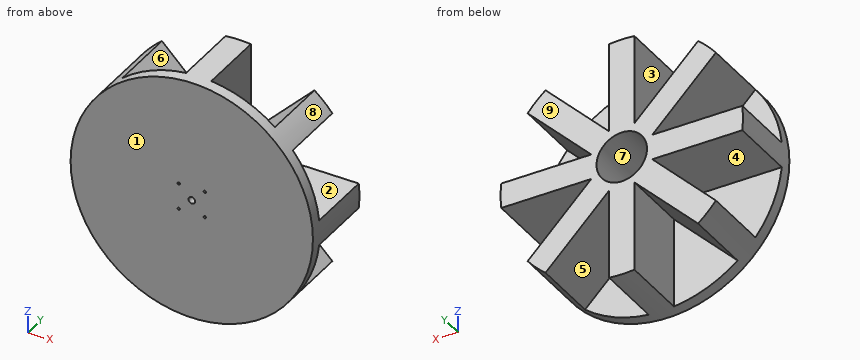
```python
from build123d import *

# Parameters (mm, degrees)
SKETCH1_R           = 144
BOSS_EXTRUDE1_DEPTH = 94
CUT_EXTRUDE1_DEPTH  = 80
SKETCH3_R           = 4
CUT_EXTRUDE2_DEPTH  = 20
CUT_EXTRUDE3_REACH  = 96
SKETCH4_R           = 1.4
SKETCH5_R           = 30
CUT_EXTRUDE4_DEPTH  = 80


with BuildPart() as part:
    # Sketch1 → Boss-Extrude1 (new body)
    with BuildSketch(Plane(origin=(0, 0, 0), x_dir=(1, 0, 0), z_dir=(0, 1, 0))):
        Circle(SKETCH1_R)
    extrude(amount=BOSS_EXTRUDE1_DEPTH)

    # Sketch2 → Cut-Extrude1 (cut)
    with BuildSketch(Plane(origin=(0, 94, 0), x_dir=(1, 0, 0), z_dir=(0, 1, 0))):
        with BuildLine():
            Line((-15, 36.213203436), (-15, 143.216619147))
            ThreePointArc((-15, 143.216619147), (-55.106414261, 133.038652682), (-90.66284086, 111.876044296))
            Line((-90.66284086, 111.876044296), (-15, 36.213203436))
        make_face()
        with BuildLine():
            Line((15, 36.213203436), (90.66284086, 111.876044296))
            ThreePointArc((90.66284086, 111.876044296), (55.106414261, 133.038652682), (15, 143.216619147))
            Line((15, 143.216619147), (15, 36.213203436))
        make_face()
        with BuildLine():
            ThreePointArc((143.216619147, 15), (133.038652682, 55.106414261), (111.876044296, 90.66284086))
            Line((111.876044296, 90.66284086), (36.213203436, 15))
            Line((36.213203436, 15), (143.216619147, 15))
        make_face()
        with BuildLine():
            ThreePointArc((111.876044296, -90.66284086), (133.038652682, -55.106414261), (143.216619147, -15))
            Line((143.216619147, -15), (36.213203436, -15))
            Line((36.213203436, -15), (111.876044296, -90.66284086))
        make_face()
        with BuildLine():
            ThreePointArc((15, -143.216619147), (55.106414261, -133.038652682), (90.66284086, -111.876044296))
            Line((90.66284086, -111.876044296), (15, -36.213203436))
            Line((15, -36.213203436), (15, -143.216619147))
        make_face()
        with BuildLine():
            ThreePointArc((-90.66284086, -111.876044296), (-55.106414261, -133.038652682), (-15, -143.216619147))
            Line((-15, -143.216619147), (-15, -36.213203436))
            Line((-15, -36.213203436), (-90.66284086, -111.876044296))
        make_face()
        with BuildLine():
            Line((-36.213203436, -15), (-143.216619147, -15))
            ThreePointArc((-143.216619147, -15), (-133.038652682, -55.106414261), (-111.876044296, -90.66284086))
            Line((-111.876044296, -90.66284086), (-36.213203436, -15))
        make_face()
        with BuildLine():
            Line((-36.213203436, 15), (-111.876044296, 90.66284086))
            ThreePointArc((-111.876044296, 90.66284086), (-133.038652682, 55.106414261), (-143.216619147, 15))
            Line((-143.216619147, 15), (-36.213203436, 15))
        make_face()
    extrude(amount=-CUT_EXTRUDE1_DEPTH, mode=Mode.SUBTRACT)

    # Sketch3 → Cut-Extrude2 (cut)
    with BuildSketch(Plane.XZ):
        Circle(SKETCH3_R)
    extrude(amount=-CUT_EXTRUDE2_DEPTH, mode=Mode.SUBTRACT)

    # Sketch4 → Cut-Extrude3 (cut, up to next)
    with BuildSketch(Plane.XZ, mode=Mode.PRIVATE) as cut_extrude3_sk1:
        with Locations((15.5, -15.5)):
            Circle(SKETCH4_R)
    cut_extrude3_tool1 = extrude(cut_extrude3_sk1.sketch, amount=-CUT_EXTRUDE3_REACH, mode=Mode.PRIVATE) & part.part
    add(cut_extrude3_tool1.solids().sort_by_distance((15.5, 0, -15.5))[0], mode=Mode.SUBTRACT)
    # Sketch4 → Cut-Extrude3 (cut, up to next)
    with BuildSketch(Plane.XZ, mode=Mode.PRIVATE) as cut_extrude3_sk2:
        with Locations((15.5, 15.5)):
            Circle(SKETCH4_R)
    cut_extrude3_tool2 = extrude(cut_extrude3_sk2.sketch, amount=-CUT_EXTRUDE3_REACH, mode=Mode.PRIVATE) & part.part
    add(cut_extrude3_tool2.solids().sort_by_distance((15.5, 0, 15.5))[0], mode=Mode.SUBTRACT)
    # Sketch4 → Cut-Extrude3 (cut, up to next)
    with BuildSketch(Plane.XZ, mode=Mode.PRIVATE) as cut_extrude3_sk3:
        with Locations((-15.5, 15.5)):
            Circle(SKETCH4_R)
    cut_extrude3_tool3 = extrude(cut_extrude3_sk3.sketch, amount=-CUT_EXTRUDE3_REACH, mode=Mode.PRIVATE) & part.part
    add(cut_extrude3_tool3.solids().sort_by_distance((-15.5, 0, 15.5))[0], mode=Mode.SUBTRACT)
    # Sketch4 → Cut-Extrude3 (cut, up to next)
    with BuildSketch(Plane.XZ, mode=Mode.PRIVATE) as cut_extrude3_sk4:
        with Locations((-15.5, -15.5)):
            Circle(SKETCH4_R)
    cut_extrude3_tool4 = extrude(cut_extrude3_sk4.sketch, amount=-CUT_EXTRUDE3_REACH, mode=Mode.PRIVATE) & part.part
    add(cut_extrude3_tool4.solids().sort_by_distance((-15.5, 0, -15.5))[0], mode=Mode.SUBTRACT)

    # Sketch5 → Cut-Extrude4 (cut)
    with BuildSketch(Plane(origin=(0, 94, 0), x_dir=(1, 0, 0), z_dir=(0, 1, 0))):
        Circle(SKETCH5_R)
    extrude(amount=-CUT_EXTRUDE4_DEPTH, mode=Mode.SUBTRACT)


solid = part.part
```
Input: part model. Units: mm. Frame: model coordinates. Face numbers are marked on the shaded views. A direction names the side the tool comes from. Give positions to 0.01 mm unless a question says otherwise; leave off trailing zeros. Order: outer loops, then holes, each group sorted by start corner. A loop starts at its lowest first (then second) coordinate and runs counter-clockwise, first axis right, second up.
1. Cut plane C-C (x = -79). Return loops of the section in (y, z), and give its area (3 significant figures).
Computed:
outline: (0, -120.4) - (14, -120.4) - (14, -100.21) - (94, -100.21) - (94, -57.79) - (14, -57.79) - (14, -15) - (94, -15) - (94, 15) - (14, 15) - (14, 57.79) - (94, 57.79) - (94, 100.21) - (14, 100.21) - (14, 120.4) - (0, 120.4) - close
area: 12,600 mm2
2. Set-up query: the marked faces 1, 2, 3, 4 and 5. Return all of +Z, -Z, +X, -X, +Y, -Y with unobstructed straight access to the full face (end or side cutting, diameter ignored); none if empty.
Computed:
face 1: +Z, -Z, +X, -X, -Y
face 2: +X, +Y
face 3: +Z, +Y
face 4: -X, +Y
face 5: -Z, +Y
3. Line query: probe 1 along Z at (x, y) = (15.5, 4.25); probe 2 along Z at (x, y) = (-15, 9); probe 3 along X at (y, z) = (16, -126). Output: solid intervals per line, ascending.
Computed:
probe 1: z = -143.16 to -16.9, -14.1 to 14.1, 16.9 to 143.16
probe 2: z = -143.22 to -16.81, -14.19 to 14.19, 16.81 to 143.22
probe 3: x = -15 to 15
4. Draft query along X for the marked faces 6, 7, 8 and 9. Return one class per face: released by +X, released by -X, zero draft, split by the parting line, or undercut.
Computed:
face 6: undercut
face 7: undercut
face 8: split by the parting line
face 9: zero draft
5. Cut plane B-B (y = 86). Return loops of the section in (x, z).
Computed:
outline: (-143.22, -15) - (-36.21, -15) - (-111.88, -90.66) arc R144 ccw to (-90.66, -111.88) - (-15, -36.21) - (-15, -143.22) arc R144 ccw to (15, -143.22) - (15, -36.21) - (90.66, -111.88) arc R144 ccw to (111.88, -90.66) - (36.21, -15) - (143.22, -15) arc R144 ccw to (143.22, 15) - (36.21, 15) - (111.88, 90.66) arc R144 ccw to (90.66, 111.88) - (15, 36.21) - (15, 143.22) arc R144 ccw to (-15, 143.22) - (-15, 36.21) - (-90.66, 111.88) arc R144 ccw to (-111.88, 90.66) - (-36.21, 15) - (-143.22, 15) arc R144 ccw to start; hole circle Ø60 at (0, 0)
6. Cut plane A-A (z = 0). Return loops of the section in (x, y), and give its area (3 significant figures).
Computed:
outline: (-144, 0) - (-4, 0) - (-4, 14) - (-30, 14) - (-30, 94) - (-144, 94) - close; (4, 0) - (144, 0) - (144, 94) - (30, 94) - (30, 14) - (4, 14) - close
area: 22,200 mm2
7. Pin query (flat end, axial travel): pin 1 Ø5 at (y, z) = (65.5, -20.5) entering from +X; pin 2 Ø22.5 at (x, z) = (-116, -66.5) entering from +Y; pin 3 Ø10 at (x, y) = (-85.5, 27.5) entering from +Z. Return the tip coordinate at first contact, or that it passes through.
Computed:
pin 1: stops at x = 44.21
pin 2: stops at y = 14
pin 3: stops at z = 111.71
8. Cut plane D-D (z = -83.5). Return loops of the section in (x, y).
Computed:
outline: (-117.32, 0) - (117.32, 0) - (117.32, 14) - (104.71, 14) - (104.71, 94) - (62.29, 94) - (62.29, 14) - (15, 14) - (15, 94) - (-15, 94) - (-15, 14) - (-62.29, 14) - (-62.29, 94) - (-104.71, 94) - (-104.71, 14) - (-117.32, 14) - close
